Autodesk Inventor part; units mm, degrees
ref_plane "YZ Plane" through (0, 0, 0) normal (1, 0, 0) x (0, 1, 0)
ref_plane "XZ Plane" through (0, 0, 0) normal (0, 1, 0) x (-1, 0, 0)
ref_plane "XY Plane" through (0, 0, 0) normal (0, 0, 1) x (1, 0, 0)
sketch "Sketch1" plane through (0, 0, 0) normal (0, 1, 0) x (-1, 0, 0)
  line L0 (5.7735, 10) -> (11.547, 0)
  line L1 (11.547, 0) -> (5.7735, -10)
  line L2 (5.7735, -10) -> (-5.7735, -10)
  line L3 (-5.7735, -10) -> (-11.547, 0)
  line L4 (-11.547, 0) -> (-5.7735, 10)
  line L5 (-5.7735, 10) -> (5.7735, 10)
  line L6 (10.3923, 0) -> (5.1962, -9)
  line L7 (5.1962, -9) -> (-5.1962, -9)
  line L8 (-5.1962, -9) -> (-10.3923, 0)
  line L9 (-10.3923, 0) -> (-5.1962, 9)
  line L10 (-5.1962, 9) -> (5.1962, 9)
  line L11 (5.1962, 9) -> (10.3923, 0)
  line L12 (0, 0.5) -> (11.2583, 0.5)
  line L13 (0, 0) -> (5.7735, 10)
  line L14 (0, 0) -> (-5.7735, 10)
  line L15 (11.547, 0) -> (-11.547, 0)
  line L16 (0, 0.5) -> (-11.2583, 0.5)
  line L17 (-0.5, 0) -> (-6.0235, 9.567)
  line L18 (0.5, 0) -> (-5.2735, 10)
  line L19 (-0.5, 0) -> (5.2735, 10)
  line L20 (-0.5, 0) -> (11.047, 0) construction
  line L21 (0.5, 0) -> (6.0235, 9.567)
  line L22 (0, -0.5) -> (11.2583, -0.5)
  line L23 (0, 0) -> (5.7735, -10)
  line L24 (0, 0) -> (-5.7735, -10)
  line L25 (0, -0.5) -> (-11.2583, -0.5)
  line L26 (-0.5, 0) -> (-6.0235, -9.567)
  line L27 (0.5, 0) -> (-5.2735, -10)
  line L28 (-0.5, 0) -> (5.2735, -10)
  line L29 (0.5, 0) -> (6.0235, -9.567)
  point P0 (-10.1036, 0.5)
  point P1 (-5.4462, 8.567)
  point P2 (-0.7887, 0.5)
  point P3 (10.1036, 0.5)
  point P4 (0.7887, 0.5)
  point P5 (5.4462, 8.567)
  point P6 (4.6962, -9)
  point P7 (-4.6962, -9)
  point P8 (0, -0.866)
  point P9 (-5.4462, -8.567)
  point P10 (-10.1036, -0.5)
  point P11 (-0.7887, -0.5)
  point P12 (10.1036, -0.5)
  point P13 (5.4462, -8.567)
  point P14 (0.7887, -0.5)
  point P15 (-4.6962, 9)
  point P16 (4.6962, 9)
  point P17 (0, 0.866)
  dimension "d0" = 20
  dimension "d1" = 18
  dimension "d2" = 60
extrude "Extrusion1" add sketch "Sketch1" along normal blind 1 contours L13 L10 L19 L5 | L0 L21 L11 L13 | L0 L12 L11 L21 | L19 L10 L18 L5 | L13 L12 L18 L19 L10 | L11 L21 L12 L13 | L0 L15 L11 L12 | L18 L10 L14 L5 | L13 L18 L12 | L12 L21 L18 L13 | L1 L22 L6 L15 | L11 L15 L21 L12 | L14 L9 L17 L4 | L18 L19 L16 L14 L10 | L18 L12 L16 L19 | L18 L13 L14 L19 L16 L12 | L18 L15 L13 | L1 L29 L6 L22 | L6 L22 L29 L15 | L27 L23 L15 | L29 L22 L23 L27 | L17 L9 L16 L4 | L14 L16 L17 L9 | L19 L14 L16 | L15 L19 L14 | L24 L28 L15 | L23 L27 L22 L25 L28 L24 | L1 L23 L6 L29 | L23 L22 L27 | L29 L6 L23 L22 | L16 L9 L15 L4 | L14 L19 L17 L16 | L26 L25 L8 L15 | L15 L9 L16 L17 | L28 L24 L25 L26 | L28 L25 L24 | L2 L28 L7 L23 | L23 L7 L28 L27 L22 | L27 L28 L25 L22 | L15 L8 L25 L3 | L25 L24 L8 L26 | L25 L28 L27 L7 L24 | L2 L27 L7 L28 | L25 L8 L26 L3 | L8 L24 L3 L26 | L7 L27 L2 L24
sketch "Sketch2" plane through (0, 1, 0) normal (0, 1, 0) x (1, 0, 0)
  circle A0 centre (0, 0) radius 0.5
  dimension "d5" = 1
extrude "Extrusion2" add sketch "Sketch2" along normal blind 2
sketch "Sketch3" plane through (0, 3, 0) normal (0, 1, 0) x (1, 0, 0)
  line L0 (-3.6084, -6.25) -> (-7.2169, 0)
  line L1 (-7.2169, 0) -> (-3.6084, 6.25)
  line L2 (-3.6084, 6.25) -> (3.6084, 6.25)
  line L3 (3.6084, 6.25) -> (7.2169, 0)
  line L4 (7.2169, 0) -> (3.6084, -6.25)
  line L5 (3.6084, -6.25) -> (-3.6084, -6.25)
  line L6 (-0.7887, -0.5) -> (-5.4462, -8.567)
  line L7 (-3.8584, -5.817) -> (3.1084, 6.25)
  line L8 (-5.4462, 8.567) -> (-0.7887, 0.5)
  line L9 (-3.8584, 5.817) -> (3.1084, -6.25)
  line L10 (-0.7887, 0.5) -> (-10.1036, 0.5)
  line L11 (-6.9282, 0.5) -> (6.9282, 0.5)
  line L12 (-10.1036, -0.5) -> (-0.7887, -0.5)
  line L13 (-6.9282, -0.5) -> (6.9282, -0.5)
  line L14 (0.7887, -0.5) -> (10.1036, -0.5)
  line L15 (-4.6962, -9) -> (0, -0.866)
  line L16 (-3.1084, -6.25) -> (3.8584, 5.817)
  line L17 (0, 0.866) -> (-4.6962, 9)
  line L18 (-3.1084, 6.25) -> (3.8584, -5.817)
  line L19 (-0.0006, -5.817) -> (3.8584, -5.817)
  line L20 (-0.0006, -5.817) -> (-3.8584, -5.817)
  line L21 (3.1084, -6.25) -> (6.9282, 0.5)
  line L22 (-3.1084, -6.25) -> (-6.9282, 0.5)
  line L23 (-7.2169, 0) -> (7.2169, 0)
  line L24 (-0.0006, 5.817) -> (3.8584, 5.817)
  line L25 (-0.0006, 5.817) -> (-3.8584, 5.817)
  line L26 (3.1084, 6.25) -> (6.9282, -0.5)
  line L27 (-3.1084, 6.25) -> (-6.9282, -0.5)
  point P0 (0, 0)
  point P1 (0, 0)
  point P2 (-2.8584, 5.817)
  point P3 (2.8584, 5.817)
  point P4 (-6.3623, 0.5)
  point P5 (-3.6034, 5.3753)
  point P6 (2.8584, -5.817)
  point P7 (-2.8584, -5.817)
  point P8 (-3.6034, -5.3753)
  point P9 (-6.3623, -0.5)
  point P10 (3.6034, -5.3753)
  point P11 (6.3623, -0.5)
  point P12 (6.3623, 0.5)
  point P13 (0.7887, 0.5)
  point P14 (3.6034, 5.3753)
  dimension "d8" = 12.5
extrude "Extrusion3" add sketch "Sketch3" along normal blind 1 contours L0 L20 L22 L5 | L0 L12 L22 L6 | L6 L22 L20 | L15 L20 L19 L9 L5 | L22 L20 L15 | L27 L22 L12 | L0 L23 L27 | L6 L13 L9 L15 L20 L22 | L21 L19 L4 L5 | L9 L19 L21 | L1 L22 L23 | L22 L23 L7 L12 | L27 L10 L9 L23 | L22 L10 L27 | L7 L9 L13 | L9 L16 L13 L18 L21 L19 | L21 L18 L19 | L9 L13 L16 | L1 L8 L27 L10 | L9 L11 L7 | L23 L16 L13 L9 | L7 L11 L18 L23 | L18 L21 L13 L4 | L16 L18 L13 | L25 L27 L8 | L1 L2 L27 L25 | L11 L8 L27 L25 L17 L7 | L7 L18 L11 | L18 L11 L16 | L23 L21 L13 L18 | L16 L11 L26 L23 | L26 L23 L4 | L13 L21 L26 | L27 L17 L25 | L7 L24 L26 L16 L11 L18 | L26 L11 L21 | L21 L3 L23 | L2 L7 L24 L25 L17 | L7 L26 L24 | L26 L16 L3 L11 | L26 L24 L16 | L2 L3 L24 L26
sketch "Sketch4" plane through (0, 4, 0) normal (0, 1, 0) x (1, 0, 0)
  line L0 (-2.8584, 5.817) -> (2.8584, 5.817)
  line L1 (3.3584, 5.817) -> (6.7169, 0)
  line L2 (6.7169, 0) -> (3.3584, -5.817)
  line L3 (3.3584, -5.817) -> (-3.3584, -5.817)
  line L4 (-3.3584, -5.817) -> (-6.7169, 0)
  line L5 (-6.7169, 0) -> (-3.3584, 5.817)
  line L6 (-3.3584, 5.817) -> (3.3584, 5.817)
  circle A0 centre (0, 0) radius 0.5
  line L7 (0, 0.5) -> (6.4282, 0.5)
  line L8 (6.4282, -0.5) -> (0, -0.5)
  arc A1 (0, 0.5) -> (0, -0.5) centre (0, 0) ccw
  point P0 (0, 5.817)
extrude "Extrusion4" cut sketch "Sketch4" against normal blind 1 contours L0 L6 L1 L7 A0 L8 L2 L3 L4 L5
sketch "Sketch5" plane through (0, 4, 0) normal (0, 1, 0) x (1, 0, 0)
  line L0 (3.3584, 5.817) -> (6.4282, 0.5)
  line L1 (6.2201, 0.8605) -> (6.7169, 0)
  line L2 (0, -0.5) -> (6.4282, -0.5)
  line L3 (6.7169, 0) -> (6.4282, -0.5)
  line L4 (6.4282, -0.5) -> (0, -0.5)
  circle A0 centre (0, 0) radius 0.5
  arc A1 (0, 0.5) -> (0, -0.5) centre (0, 0) ccw
  line L5 (0, 0.5) -> (6.2201, 0.8605)
extrude "Extrusion5" cut sketch "Sketch5" against normal blind 0.5
sketch "Sketch6" plane through (0, 0, 0) normal (0, -1, 0) x (1, 0, 0)
  line L0 (10.3923, 0) -> (5.1962, -9)
  line L1 (5.1962, -9) -> (-5.1962, -9)
  line L2 (-5.1962, -9) -> (-10.3923, 0)
  line L3 (-10.3923, 0) -> (-5.1962, 9)
  line L4 (-5.1962, 9) -> (5.1962, 9)
  line L5 (5.1962, 9) -> (10.3923, 0)
  line L6 (10.1036, -0.5) -> (0, -0.5)
  line L7 (0.7887, 0.5) -> (10.1036, 0.5)
  line L8 (6.4282, 0.5) -> (0, 0.5)
  line L9 (0, -0.5) -> (0, 0.5)
  line L10 (0, 0.5) -> (10.1036, 0.5)
  arc A0 (0, 0.5) -> (0, -0.5) centre (0, 0) ccw
  arc A1 (0, 0.5) -> (0, -0.5) centre (0, 0) ccw
  dimension "d15" = 18
extrude "Extrusion6" cut sketch "Sketch6" against normal blind 1 contours L0 L1 L2 L3 L4 L5 L7 L8 A0 L6
sketch "Sketch7" plane through (0, 0, 0) normal (0, -1, 0) x (1, 0, 0)
  line L0 (10.1036, 0.5) -> (5.1962, 9)
  line L1 (9.7836, 1.0542) -> (10.3923, 0)
  line L2 (10.3923, 0) -> (10.1036, -0.5)
  line L3 (10.1036, -0.5) -> (0, -0.5)
  arc A0 (0, 0.5) -> (0, -0.5) centre (0, 0) ccw
  line L4 (0, 0.5) -> (9.7836, 1.0542)
  point P0 (0, 0)
extrude "Extrusion7" cut sketch "Sketch7" against normal blind 0.5
sketch "Sketch8" plane through (-7.2169, 3, 0) normal (-0.866, 0, -0.5) x (-0.5, 0, 0.866)
  line L0 (-4.0415, 0.5) -> (-3.1084, 0.5)
  circle A0 centre (-3.6084, 0.5) radius 0.5022
  point P0 (-3.6084, -3)
  point P1 (-3.1754, 0.5)
Read the model definition and answer for the solid it produces. Units are mm, in the model's axes. A direction names the side the tool comes from. Round coordinates to 2 decimals unless told otherwise and drop trailing zeros. Write each loop counter-clockwise with the first axis right and the second up, starting at its lowest first coordinate (ties: lowest second). Pieces come first, ordered by that corner, then holes. Notation, with made-up numbers: (-31.5, 8.5) - (26.5, 8.5) arc R22 cw to (26.5, 31.5) - close; hole circle Ø2 at (4, -20.5). An arc over 180 degrees is marked (long way). Use a Markdown table: item, result.
(1) Each of these flat-tipped pins is pushed along its axis until it touches: pin 1 Ø0.6 at (x, y) = (2, 3) entering from -Z; pin 2 Ø1.1 at (x, y) = (0.5, 3.5) entering from +Z; pin 3 Ø0.8 at (x, z) = (4, 0) entering from +Y; pin 4 Ø8 at (x, z) = (4.5, 1.5) entering from +Y. Where does it stop, or does it pass through?
Reported:
| item | result |
|---|---|
| pin 1 | z = -6.25 |
| pin 2 | z = 6.25 |
| pin 3 | y = 3.5 |
| pin 4 | y = 4 |
(2) Straight lines are drawn through the part: line 1 along Z through (x, y) = (0.75, 3.25); line 2 along Y through (x, z) = (10.5, -0.75); line 3 along X through (y, z) = (0.8, 8). For each, find the intervals that lie inside material, in ascending order. Write a range as [from, to].
Reported:
| item | result |
|---|---|
| line 1 | [-6.25, -5.82], [-0.5, 0.5], [5.82, 6.25] |
| line 2 | [0, 1] |
| line 3 | [-6.93, -5.77], [5.77, 6.93] |
(3) The mould has two halves that part along X. Classify faces 1 (the flat face through (8.7, 0.49, 4.93)), 2 (the flat face through (5, 0.5, 0)), 3 (the flat face through (-5.387, 3.493, 3.169)): released by +X, released by -X, zero draft, split by the parting line, or undercut.
Reported:
| item | result |
|---|---|
| face 1 | released by +X |
| face 2 | undercut |
| face 3 | released by -X |
(4) The part is cut by section A-A (z = -6.5). Write down the section's boundary in (x, y).
Reported:
| item | result |
|---|---|
| outline | (-7.79, 0) - (-6.64, 0) - (-6.64, 1) - (-7.79, 1) - close; (6.64, 0) - (7.79, 0) - (7.79, 1) - (6.64, 1) - close |
(5) Which of the six approach directions +Z, -Z, +X, -X, +Y, -Y give full straight-line access (tool end or side, diameter ignored) to faces 4 (the flat face through (8.62, 0.49, -5.07)), 5 (the flat face through (3, 3.5, 0)), 6 (the flat face through (0.1, 0.5, 9))?
Reported:
| item | result |
|---|---|
| face 4 | -Z, +X, +Y, -Y |
| face 5 | +Y |
| face 6 | +Y, -Y |
(6) The part is cut by section C-C (x = -6.25). Write down the section's boundary in (y, z), then the cut area to 3 significant figures.
Reported:
| item | result |
|---|---|
| outline | (0, -9.17) - (1, -9.17) - (1, -7.17) - (0, -7.17) - close; (0, 7.17) - (1, 7.17) - (1, 9.17) - (0, 9.17) - close; (3, -1.67) - (4, -1.67) - (4, -0.81) - (3, -0.81) - close; (3, 0.81) - (4, 0.81) - (4, 1.67) - (3, 1.67) - close |
| area | 5.73 mm2 |
(7) The part is cut by section B-B (x = 7.75). Write down the section's boundary in (y, z).
Reported:
| item | result |
|---|---|
| outline | (0, -6.58) - (1, -6.58) - (1, -4.58) - (0, -4.58) - close; (0, 4.58) - (1, 4.58) - (1, 6.58) - (0, 6.58) - close; (0.5, -0.5) - (1, -0.5) - (1, 0.5) - (0.5, 0.5) - close |
(8) The part is cut by section D-D (y = 1.45). Write down the section's boundary in (x, z).
Reported:
| item | result |
|---|---|
| outline | circle Ø1 at (0, 0) |
